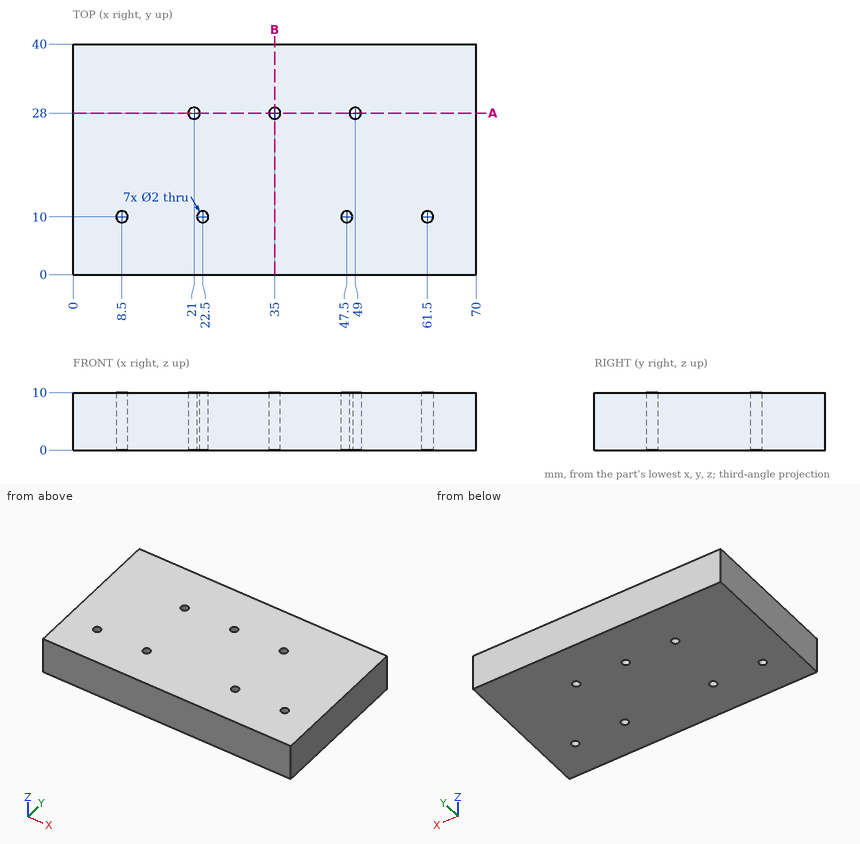
Job drawing, mm, ordinate dimensions from the low corner. One solid piece. Give positions to 0.01 mm unless a question says otherwise; leave off trailing zeros. Write each loop counter-clockwise with the first axis right and the second up, starting at its lowest first coordinate (ties: lowest second). Pieces come first, ordered by that corner, then holes. Notation, with made-up numbers: (-31.75, -26) -> (-26.75, -26) arc R16 ccw to (-26.75, -2) -> close; hole circle Ø11 at (44.25, 20). An arc over 180 degrees is marked (long way). Return JSON: item names as keys, results as strings.
Item 1: Band-saw the part on A-A (y = 28). List the corners of the cut face in (x, z).
Answer below:
{"outline": "(0, 0) -> (20, 0) -> (20, 10) -> (0, 10) -> close; (22, 0) -> (34, 0) -> (34, 10) -> (22, 10) -> close; (36, 0) -> (48, 0) -> (48, 10) -> (36, 10) -> close; (50, 0) -> (70, 0) -> (70, 10) -> (50, 10) -> close"}
Item 2: Band-saw the part on B-B (x = 35). List the corners of the cut face in (y, z), then the cut area to 3 significant figures.
Answer below:
{"outline": "(0, 0) -> (27, 0) -> (27, 10) -> (0, 10) -> close; (29, 0) -> (40, 0) -> (40, 10) -> (29, 10) -> close", "area": "380 mm2"}
Item 3: Drill centre lines: probe 1 along Y at (x, z) = (35, 6); probe 2 along Y at (x, z) = (47.5, 2.75). Where is each one in solid material? Low to high.
Answer below:
{"probe 1": "y = 0 to 27, 29 to 40", "probe 2": "y = 0 to 9, 11 to 40"}
